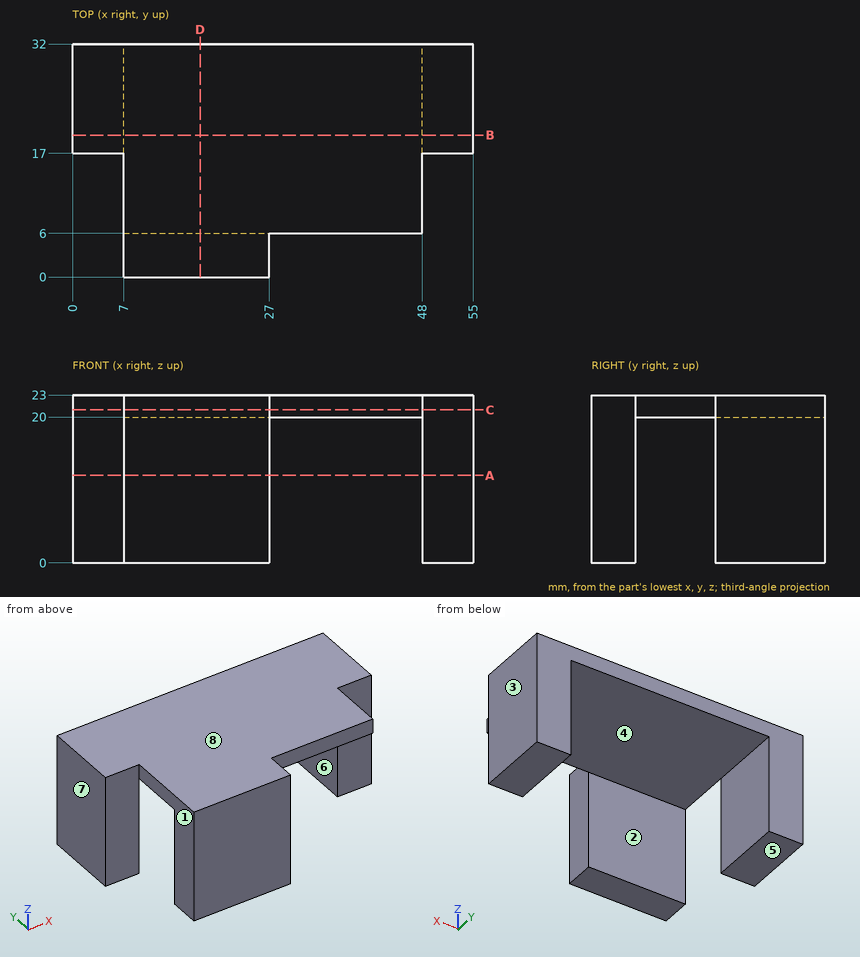
Design review of the part shown in the three views and the two pictorial views. Dimensions are in mm from the part's minimum x, y and z. A direction names the side the tool comes from. Round coordinates to 2 decimals unless told otherwise and drop trailing zeros. Order: outer loops, then holes, each group sorted by start corner. A loop starts at its lowest first (then second) coordinate and runs counter-clockwise, first axis right, second up. Notation, with made-up numbers: M 37.5,17 L 42.5,17 A22 cw 42.5,26 Z; hole C 81.25,-1 d9. An arc over 180 degrees is marked long. Put each result on its own line as item: value.
Q1. Draft analysis for pull direction X (two halves, no side actions). For the marked faces 6, 7 and 8, state which applies: released by +X, released by -X, zero draft, split by the parting line, or undercut.
Reported:
face 6: undercut
face 7: released by -X
face 8: zero draft
Q2. Consider section B-B (y = 19.5). State the section outline as (x, z) points.
Reported:
outline: M 0,0 L 7,0 L 7,20 L 48,20 L 48,0 L 55,0 L 55,23 L 0,23 Z
Q3. To check wall thickness, follow line 1 (X direction, y = 23, z = 18.5); line 2 (X direction, y = 5.5, z = 21.5); line 3 (Z direction, x = 14.5, y = 22.5). State the ranges of each line that lie inside material, in increasing order.
Reported:
line 1: 0 to 7, 48 to 55
line 2: 7 to 27
line 3: 20 to 23
Q4. Consider section D-D (x = 17.5). State the section outline as (y, z) points, and give its area (3 significant figures).
Reported:
outline: M 0,0 L 6,0 L 6,20 L 32,20 L 32,23 L 0,23 Z
area: 216 mm²
Q5. Insertion check: pin 1 Ø3 at (x, z) = (23.5, 19) entering from +Y; pin 2 Ø13.5 at (y, z) = (8.5, 6) entering from -X; pin 3 Ø8 at (x, z) = (40.5, 14) entering from -Y; pin 4 Ø5.5 at (x, z) = (52.5, 16) entering from -Y. Each pin has a flat end and moves straight along its axis. Give the tip position at first contact, or say it passes through.
Reported:
pin 1: y = 32
pin 2: x = 7
pin 3: through
pin 4: y = 17
Q6. Consider section C-C (z = 21). State the section outline as (x, y) points.
Reported:
outline: M 0,17 L 7,17 L 7,0 L 27,0 L 27,6 L 48,6 L 48,17 L 55,17 L 55,32 L 0,32 Z
Q7. Consider section A-A (z = 12). State the section outline as (x, y) points, and give its area (3 significant figures).
Reported:
outline: M 0,17 L 7,17 L 7,32 L 0,32 Z; M 7,0 L 27,0 L 27,6 L 7,6 Z; M 48,17 L 55,17 L 55,32 L 48,32 Z
area: 330 mm²
Q8. Machinability: for the marked faces 1, 2, 3, 4 and 5, which of the approach directions +Z, -Z, +X, -X, +Y, -Y give a long, thin tool a straight path to every point of the face, cutting with its end or side? Answer none if there is none.
Reported:
face 1: +Z, -Z, -X, -Y
face 2: -Z, +X, -X, +Y
face 3: +Z, -Z, +X, +Y, -Y
face 4: -Z, +Y
face 5: -Z, +X, -X, +Y, -Y
